from build123d import *
from build123d.topology import SkipClean

# Parameters (mm, degrees)
SKETCH_1_R      = 16.35
EXTRUDE_1_DEPTH = 9
SKETCH_2_R      = 17.29
EXTRUDE_2_DEPTH = 6
SKETCH_3_R      = 5.5
SKETCH_3_R_2    = 1.9
SKETCH_3_R_3    = 2.65
EXTRUDE_3_DEPTH = 4
EXTRUDE_4_DEPTH = 7.7


with BuildPart() as part:
    # 草图1 → 凸台-拉伸1 (new body)
    with BuildSketch(Plane(origin=(0, 0, 0), x_dir=(1, 0, 0), z_dir=(0, 1, 0))):
        with Locations(Location((0, 0, 0), (0, 0, 270))):
            Circle(SKETCH_1_R)
    extrude(amount=EXTRUDE_1_DEPTH)

    # 草图2 → 凸台-拉伸2 (add)
    with BuildSketch(Plane.XZ):
        with Locations(Location((0, 0, 0), (0, 0, 270))):
            Circle(SKETCH_2_R)
    extrude(amount=EXTRUDE_2_DEPTH)

    # 草图3 → 凸台-拉伸3 (add)
    with BuildSketch(Plane.XZ.offset(6)):
        with Locations(Location((0, 0, 0), (0, 0, 270))):
            Circle(SKETCH_3_R)
        with Locations(Location((-6.6, -9.56, 0), (0, 0, 270))):
            Circle(SKETCH_3_R_2)
        with Locations(Location((-10, 5.68, 0), (0, 0, 270))):
            Circle(SKETCH_3_R_3)
        with Locations(Location((6.6, -9.56, 0), (0, 0, 90))):
            Circle(SKETCH_3_R_2)
        with Locations(Location((10, 5.68, 0), (0, 0, 90))):
            Circle(SKETCH_3_R_3)
    extrude(amount=EXTRUDE_3_DEPTH)

    # 草图4 → 凸台-拉伸4 (add)
    with SkipClean():  # the faces are left unmerged after this step: merging them gives an invalid solid
        with BuildSketch(Plane.XZ.offset(10)):
            with BuildLine():
                Line((-12.309220648, 6.98), (-7.690779352, 6.98))
                ThreePointArc((-7.690779352, 6.98), (-7.35, 5.68), (-7.690779352, 4.38))
                Line((-7.690779352, 4.38), (-12.309220648, 4.38))
                ThreePointArc((-12.309220648, 4.38), (-12.65, 5.68), (-12.309220648, 6.98))
            make_face()
            with BuildLine():
                Line((12.309220648, 6.98), (7.690779352, 6.98))
                ThreePointArc((7.690779352, 6.98), (7.35, 5.68), (7.690779352, 4.38))
                Line((7.690779352, 4.38), (12.309220648, 4.38))
                ThreePointArc((12.309220648, 4.38), (12.65, 5.68), (12.309220648, 6.98))
            make_face()
        extrude(amount=EXTRUDE_4_DEPTH)


solid = part.part
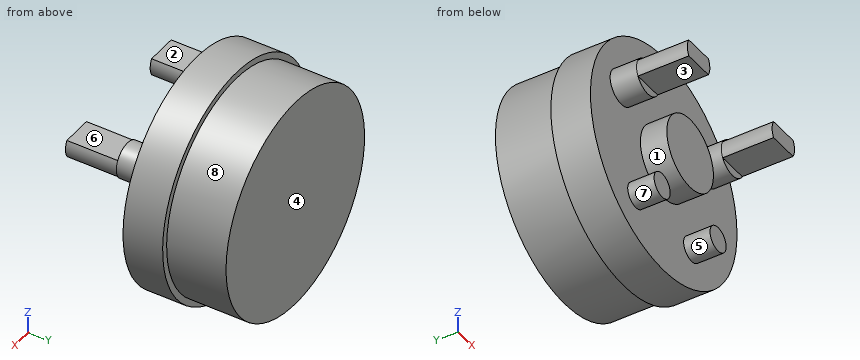
Part model, mm, in its own coordinate system. Face numbers are marked on the shaded views. A direction names the side the tool comes from. Give positions to 0.01 mm unless a question says otherwise; leave off trailing zeros. Order: outer loops, then holes, each group sorted by start corner. A loop starts at its lowest first (then second) coordinate and runs counter-clockwise, first axis right, second up. Notation, with made-up numbers: (55, 37) - (104, 37) arc R22 cw to (104, 56) - close; hole circle Ø1 at (68.25, 80.25). An arc over 180 degrees is marked (long way). Use a Markdown table: item, result.
1) Two-plate mould, pull along Z, no slides. Class the marked faces 5, 6, 7 and 8: +Z half, -Z half, draft (parallel to the pull), parting line (faces both ways), or undercut.
Checked values:
| item | result |
|---|---|
| face 5 | undercut |
| face 6 | +Z half |
| face 7 | undercut |
| face 8 | parting line |
2) Saw through at B-B on x = 0. List the corners of the cut face in (y, z), plus the area to 3 significant figures.
Checked values:
| item | result |
|---|---|
| outline | (-10, -5.5) - (-6, -5.5) - (-6, -17.29) - (0, -17.29) - (0, -16.35) - (9, -16.35) - (9, 16.35) - (0, 16.35) - (0, 17.29) - (-6, 17.29) - (-6, 5.5) - (-10, 5.5) - close |
| area | 546 mm² |
3) Flat gauge pins, fed straight in: P1, Ø1.1, axis at x = -6, z = -10.5, coming from the -Y side; P2, Ø2, axis at y = -3, z = -11.5, coming from the +X side; P3, Ø6, axis at y = 1, z = -12.5, coming from the -X side. Where does each tip first touch, or does it go through?
Checked values:
| item | result |
|---|---|
| P1 | y = -10 |
| P2 | x = 13.74 |
| P3 | x = -14.33 |
4) 3-axis set-ups, long thin cutter, end or side, ignore diameter. For the marked faces 1, 2, 3 and 4: which of +Z, -Z, +X, -X, +Y, -Y reach the whole face in a straight line?
Checked values:
| item | result |
|---|---|
| face 1 | -Y |
| face 2 | +Z, +X, -X, -Y |
| face 3 | -Z, +X, -X, -Y |
| face 4 | +Z, -Z, +X, -X, +Y |
5) Probe L1, parallel to Y at x = 13, z = -0.5; L2, parallel to Y at x = 0, z = -5; L3, parallel to Z at x = -8, y = -12.5. List the from-to ranges inside material, lowest first. Write a range as from..to.
Checked values:
| item | result |
|---|---|
| L1 | -6..9 |
| L2 | -10..9 |
| L3 | 4.38..6.98 |
6) Saw through at A-A on y = -8.25. List the corners of the cut face in (x, z).
Checked values:
| item | result |
|---|---|
| outline | circle Ø5.3 at (-10, 5.68); circle Ø3.8 at (-6.6, -9.56); circle Ø11 at (0, 0); circle Ø3.8 at (6.6, -9.56); circle Ø5.3 at (10, 5.68) |
7) Saw through at C-C on z = 0. List the corners of the cut face in (x, y), plus the area to 3 significant figures.
Checked values:
| item | result |
|---|---|
| outline | (-17.29, -6) - (-5.5, -6) - (-5.5, -10) - (5.5, -10) - (5.5, -6) - (17.29, -6) - (17.29, 0) - (16.35, 0) - (16.35, 9) - (-16.35, 9) - (-16.35, 0) - (-17.29, 0) - close |
| area | 546 mm² |
8) Saw through at D-D on y = 4.5. List the corners of the cut face in (x, z), plus the area to 3 significant figures.
Checked values:
| item | result |
|---|---|
| outline | circle Ø32.7 at (0, 0) |
| area | 840 mm² |
